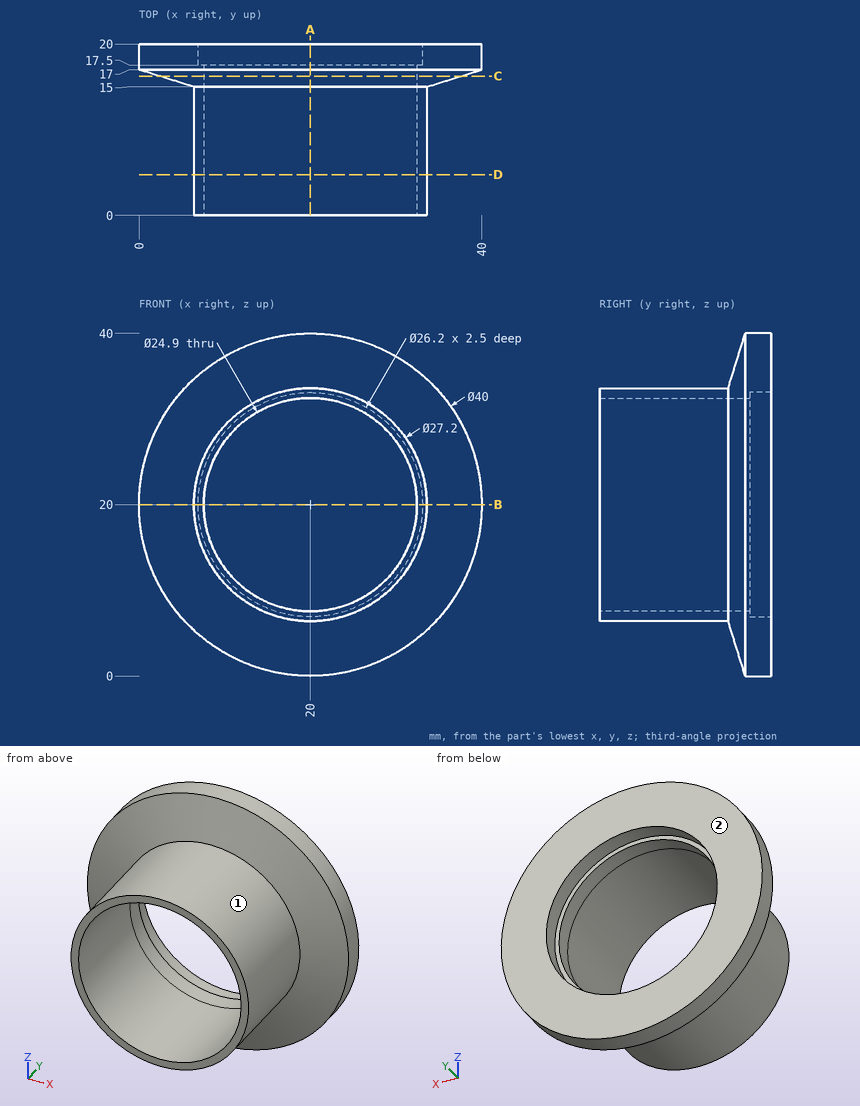
Check sheet for the drawn part. Datum: minimum x, y, z corner. Units: mm. A direction names the side the tool comes from. Coordinates: 2 decimals unless noted, no trailing zeros. Write each loop counter-clockwise with the first axis right and the second up, starting at its lowest first coordinate (ties: lowest second). Pieces come first, ordered by that corner, then holes. Notation, with made-up numbers: M 86,25 L 139,25 A16 cw 139,37 Z; hole C -33,24.25 d11. An arc over 180 degrees is marked long. Use a Markdown table: item, result.
Q1. Set-up check for the marked faces 1 and 2: record each of +Z, -Z, +X, -X, +Y, -Y from which the full face is reachable in a straight line by a thin tool's end or side.
Reply:
| item | result |
|---|---|
| face 1 | -Y |
| face 2 | +Z, -Z, +X, -X, +Y |
Q2. Sectioned sample at D-D, the plane y = 4.75. Record the boundary of the cut face in (x, z), plus the area to 3 significant figures.
Reply:
| item | result |
|---|---|
| outline | C 20,20 d27.2; hole C 20,20 d24.9 |
| area | 94.1 mm² |
Q3. Sectioned sample at A-A, the plane x = 20. Record the boundary of the cut face in (y, z).
Reply:
| item | result |
|---|---|
| outline | M 0,6.4 L 15,6.4 L 17,0 L 20,0 L 20,6.9 L 17.5,6.9 L 17.5,7.55 L 0,7.55 Z; M 0,32.45 L 17.5,32.45 L 17.5,33.1 L 20,33.1 L 20,40 L 17,40 L 15,33.6 L 0,33.6 Z |
Q4. Thickness scan on line 1 (X direction, y = 18.55, z = 20); line 2 (X direction, y = 4.75, z = 20). Record the ranges inside material, lowest first.
Reply:
| item | result |
|---|---|
| line 1 | x = 0 to 6.9, 33.1 to 40 |
| line 2 | x = 6.4 to 7.55, 32.45 to 33.6 |
Q5. Go/stop test with flat-tipped pins: P1, Ø13, axis at x = 18.5, z = 14, coming from the +Y side; P2, Ø4, axis at y = 3.5, z = 9, coming from the +X side; P3, Ø5, axis at x = 20, z = 7.5, coming from the +Y side; P4, Ø8, axis at x = 32.5, y = 14, coming from the +Z side. Record where each tip stops, or that it passes through.
Reply:
| item | result |
|---|---|
| P1 | stops at y = 17.5 |
| P2 | stops at x = 30.2 |
| P3 | stops at y = 20 |
| P4 | stops at z = 37.4 |
Q6. Sectioned sample at C-C, the plane y = 16.25. Record the boundary of the cut face in (x, z), plus the area to 3 significant figures.
Reply:
| item | result |
|---|---|
| outline | C 20,20 d35.2; hole C 20,20 d24.9 |
| area | 486 mm² |
Q7. Sectioned sample at B-B, the plane z = 20. Record the boundary of the cut face in (x, y).
Reply:
| item | result |
|---|---|
| outline | M 0,17 L 6.4,15 L 6.4,0 L 7.55,0 L 7.55,17.5 L 6.9,17.5 L 6.9,20 L 0,20 Z; M 32.45,0 L 33.6,0 L 33.6,15 L 40,17 L 40,20 L 33.1,20 L 33.1,17.5 L 32.45,17.5 Z |
